Autodesk Inventor part; units mm, degrees
ref_plane "YZ Plane" through (0, 0, 0) normal (1, 0, 0) x (0, 1, 0)
ref_plane "XZ Plane" through (0, 0, 0) normal (0, 1, 0) x (-1, 0, 0)
ref_plane "XY Plane" through (0, 0, 0) normal (0, 0, 1) x (1, 0, 0)
sketch "Sketch1" plane through (0, 0, 0) normal (0, 1, 0) x (-1, 0, 0)
  circle A0 centre (0, 0) radius 2.8
  circle A1 centre (0, 0) radius 7.5
  dimension "d0" = 5.6
  dimension "d1" = 15
extrude "Extrusion1" add sketch "Sketch1" along normal blind 14.75
sketch "Sketch2" plane through (0, 14.75, 0) normal (0, 1, 0) x (1, 0, 0)
  circle A0 centre (0, 0) radius 4.5
  circle A1 centre (0, 0) radius 2.8
  dimension "d4" = 9
extrude "Extrusion2" add sketch "Sketch2" along normal blind 0.75
chamfer "Chamfer1" distance 1 angle 45 1 edges at (7.5, 14.75, 0)
properties part number "x carraige sliding spacer long" material "ABS Plastic"
The model under review builds one solid part; all positions refer to its coordinate system, in mm. A direction names the side the tool comes from. Give positions to 0.01 mm unless a question says otherwise; leave off trailing zeros. Loops run counter-clockwise (first coordinate to the right, second up) from the corner with the lowest first, then second, coordinate; pieces in that order, holes last. Notation, with made-up numbers: (-7, -33.5) -> (14, -33.5) arc R33 cw to (14, -2.5) -> close; hole circle Ø5 at (-25, 2.5). An arc over 180 degrees is marked (long way). Put each result on its own line as item: value. Start each with the question number.
1. We need section B-B on y = 5.5. State the section outline as (x, z) points.
2. For faces 1 (the face through (0, 0, -3)), 2 (the face through (1.54, 14.75, 4.42)), list the 3-axis set-ups (+Z, -Z, +X, -X, +Y, -Y) from which the entire face can be reached by the end or side of a thin tool; tool diameter is ignored.
3. Clearance check with flat-ended pins moving along their axes: P1, Ø4.5, axis at x = 0, z = 0, coming from the +Y side; P2, Ø4, axis at y = 13, z = -2.5, coming from the -X side; P3, Ø2, axis at y = 14, z = 6, coming from the +X side; P4, Ø1.5, axis at x = 1.5, y = 7.5, coming from the -Z side. State where each tip first meets the part, or that it passes through.
4. Wall thickness on probe 1 along Z at (x, y) = (0, 8); probe 2 along Y at (x, z) = (-1.25, -6); probe 3 along Z at (x, y) = (2.25, 14.25): over which ranges is each line inside the solid? List them lowest first.
Determined:
1. outline: circle Ø15 at (0, 0); hole circle Ø5.6 at (0, 0)
2. face 1: +Z, -Z, +X, -X, -Y
2. face 2: +Y
3. P1: through
3. P2: x = -7.48
3. P3: x = 5.56
3. P4: z = -7.46
4. probe 1: -7.5 to -2.8, 2.8 to 7.5
4. probe 2: 0 to 14.75
4. probe 3: -6.63 to -1.67, 1.67 to 6.63
